Geometry: final body of the model. Coordinates: model frame, mm. Coordinates: 2 decimals unless noted, no trailing zeros. Write each loop counter-clockwise with the first axis right and the second up, starting at its lowest first coordinate (ties: lowest second). Pieces come first, ordered by that corner, then holes. Notation, with made-up numbers: M 23.5,7.25 L 43.5,7.25 A11 ccw 43.5,26.25 Z; hole C 11,67.25 d4. An arc over 180 degrees is marked long. Write item = value, one per line. Start each with the question number.
Item 1: Pull-direction query (Y, two-part tool) for faces 1 (the flat face through (1, -18, 25.4)), 2 (the cylindrical face through (-0.023, 1.016, 12.522)); classes: +Y half, -Y half, draft (parallel to the pull), parting line (faces both ways), or undercut.
Item 2: Section A-A on z = 17.5. Output: boundary loops of the cut face in (x, y).
Item 3: First-contact query: pin 1 Ø3 at (y, z) = (-31.5, 18.5) entering from -X; pin 2 Ø1 at (y, z) = (-2.5, 20.5) entering from +X; pin 3 Ø6 at (y, z) = (-30.5, 6.5) entering from -X. Flat tips, straight axial feed; report the tip coordinate or a pass-through.
Item 4: Section B-B on y = -9. Output: boundary loops of the cut face in (x, z), plus the area to 3 significant figures.
Item 5: Section C-C on y = -13.5. Output: boundary loops of the cut face in (x, z).
Item 6: Ray query, L1, parallel to X at y = -33, z = 2.75; L2, parallel to X at y = -25, z = 3.75; L3, parallel to Y at x = 0, z = 10.5. Return the intervals inside material, ascending. Write a range as [from, to].
from build123d import *

# Parameters (mm, degrees)
F1_DEPTH = 25.4
F2_W     = 9.525
F2_H     = 22.225
F3_DEPTH = 0.254


with BuildPart() as f1:
    # F0 (on Top) → F1 (new body)
    with BuildSketch(Plane.XY):
        with BuildLine():
            ThreePointArc((-1.015796583, -0.020329831), (0, 1.016), (1.015796583, -0.020329831))
            Line((1.015796583, -0.020329831), (0.254, -38.0841173196))
            ThreePointArc((0.254, -38.0841173196), (0.4752066949, -38.6499228834), (1.0317084, -38.8935910804))
            Line((1.0317084, -38.8935910804), (1.8093876634, -0.0362125114))
            ThreePointArc((1.8093876634, -0.0362125114), (0, 1.80975), (-1.8093876634, -0.0362125114))
            Line((-1.8093876634, -0.0362125114), (-1.0317084, -38.8935910804))
            ThreePointArc((-1.0317084, -38.8935910804), (-0.4752066949, -38.6499228834), (-0.254, -38.0841173196))
            Line((-0.254, -38.0841173196), (-1.015796583, -0.020329831))
        make_face()
    extrude(amount=F1_DEPTH)

    # F2 (on face) → F3 (cut)
    with BuildSketch(Plane(origin=(1.8093876634, -0.0362125114, 0), x_dir=(0.0200096762, 0.9997997864, 0), z_dir=(0.9997997864, -0.0200096762, 0))):
        with Locations((-5.55625, 12.7)):
            Rectangle(F2_W, F2_H)
    extrude(amount=-F3_DEPTH, mode=Mode.SUBTRACT)


solid = f1.part
Responses:
q1.face_1 = draft
q1.face_2 = undercut
q2.outline = M -1.81,-0.04 L -1.03,-38.89 A0.79 ccw -0.25,-38.08 L -1.02,-0.02 A1.02 cw long 1.02,-0.02 L 0.25,-38.08 A0.79 ccw 1.03,-38.89 L 1.6,-10.35 L 1.35,-10.35 L 1.54,-0.82 L 1.79,-0.83 L 1.81,-0.04 A1.81 ccw long Z
q3.pin_1 = -1.21
q3.pin_2 = 1.52
q3.pin_3 = -1.26
q4.outline = M -1.63,0 L -0.84,0 L -0.84,25.4 L -1.63,25.4 Z; M 0.84,0 L 1.63,0 L 1.63,1.59 L 1.38,1.59 L 1.38,23.81 L 1.63,23.81 L 1.63,25.4 L 0.84,25.4 Z
q4.area = 34.7 mm²
q5.outline = M -1.54,0 L -0.75,0 L -0.75,25.4 L -1.54,25.4 Z; M 0.75,0 L 1.54,0 L 1.54,25.4 L 0.75,25.4 Z
q6.L1 = [-1.15, -0.36], [0.36, 1.15]
q6.L2 = [-1.31, -0.52], [0.52, 1.31]
q6.L3 = [1.02, 1.81]
